The model under review builds one solid part; all positions refer to its coordinate system, in mm. Round coordinates to 2 decimals unless told otherwise and drop trailing zeros. Loops run counter-clockwise (first coordinate to the right, second up) from the corner with the lowest first, then second, coordinate; pieces in that order, holes last. Notation, with made-up numbers: M -27,22.5 L 26,22.5 A31 cw 26,55.5 Z; hole C -6.5,-2.5 d1. An arc over 180 degrees is marked long. One line per question, with ' | ' between items.
Autodesk Inventor part; units mm, degrees
ref_plane "YZ Plane" through (0, 0, 0) normal (1, 0, 0) x (0, 1, 0)
ref_plane "XZ Plane" through (0, 0, 0) normal (0, 1, 0) x (-1, 0, 0)
ref_plane "XY Plane" through (0, 0, 0) normal (0, 0, 1) x (1, 0, 0)
sketch "スケッチ1" plane through (0, 0, 0) normal (0, 0, 1) x (1, 0, 0)
  circle A0 centre (0, 0) radius 32
  dimension "d0" = 64
extrude "押し出し1" add sketch "スケッチ1" along normal blind 2
sketch "スケッチ2" plane through (0, 0, 2) normal (0, 0, 1) x (1, 0, 0)
  circle A0 centre (-15, 0) radius 1.6
  circle A1 centre (15, 0) radius 1.6
  point P0 (0, 0)
  dimension "d3" = 3.2
  dimension "d4" = 3.2
  dimension "d5" = 15
  dimension "d6" = 15
hole "穴1" at (-15, 0, 2) at (15, 0, 2) direction (0, 0, -1) diameter 3.2 depth 2
sketch "スケッチ3" plane through (0, 0, 2) normal (0, 0, 1) x (1, 0, 0)
  circle A0 centre (0, 0) radius 4
  dimension "d14" = 8
extrude "押し出し2" cut sketch "スケッチ3" against normal blind 2
equation "\"BendRadius\" = Thickness"
equation "\"BendReliefWidth\" = Thickness"
equation "\"BendReliefDepth\" = 0.5 * Thickness"
equation "\"CornerReliefSize\" = 4 * Thickness"
equation "\"MinimumRemnant\" = 2 * Thickness"
equation "\"TransitionRadius\" = BendRadius"
equation "\"JacobiRadiusSize\" = BendRadius"
equation "\"GapSize\" = Thickness"
properties part number "nhk34"
1) Add section A-A on y = 0. State the section outline as (x, z) points, then the cut area to 3 significant figures.
Output values:
outline: M -32,0 L -16.6,0 L -16.6,2 L -32,2 Z; M -13.4,0 L -4,0 L -4,2 L -13.4,2 Z; M 4,0 L 13.4,0 L 13.4,2 L 4,2 Z; M 16.6,0 L 32,0 L 32,2 L 16.6,2 Z | area: 99.2 mm²
2) Add section B-B on x = -0.5. State the section outline as (y, z) points, then the cut area to 3 significant figures.
Output values:
outline: M -32,0 L -3.97,0 L -3.97,2 L -32,2 Z; M 3.97,0 L 32,0 L 32,2 L 3.97,2 Z | area: 112 mm²
3) Mouldability with a two-part tool opening along Y and no side actions: class faces 1 (the flat face through (0, -7, 0)), 2 (the cylindrical face through (-6.94, 31.24, 0.99)), 3 (the cylindrical face through (-16.586, 0.208, 0.986)), 4 (the cylindrical face through (13.414, 0.208, 0.986)) as +Y half, -Y half, draft (parallel to the pull), parting line (faces both ways), or undercut.
Output values:
face 1: draft | face 2: parting line | face 3: undercut | face 4: undercut
4) Insertion check: P1, Ø3.5, axis at x = -15, y = 0, coming from the -Z side; P2, Ø6.5, axis at x = 0, y = 0, coming from the +Z side. Each pin has a flat end and moves straight along its axis. Give the tip position at first contact, or say it passes through.
Output values:
P1: stops at z = 0 | P2: passes through
5) For line 1 (Y direction, x = 0, z = 0.85); line 2 (X direction, y = -2, z = 1.3); line 3 (Y direction, x = -15, z = 1.15), list the stretches that pass through material, from the lowest coordinate up.
Output values:
line 1: y = -32 to -4, 4 to 32 | line 2: x = -31.94 to -3.46, 3.46 to 31.94 | line 3: y = -28.27 to -1.6, 1.6 to 28.27
6) Add section D-D on x = 15. State the section outline as (y, z) points.
Output values:
outline: M -28.27,0 L -1.6,0 L -1.6,2 L -28.27,2 Z; M 1.6,0 L 28.27,0 L 28.27,2 L 1.6,2 Z
7) Add section C-C on z = 1.55. State the section outline as (x, y) points.
Output values:
outline: C 0,0 d64; hole C -15,0 d3.2; hole C 0,0 d8; hole C 15,0 d3.2
